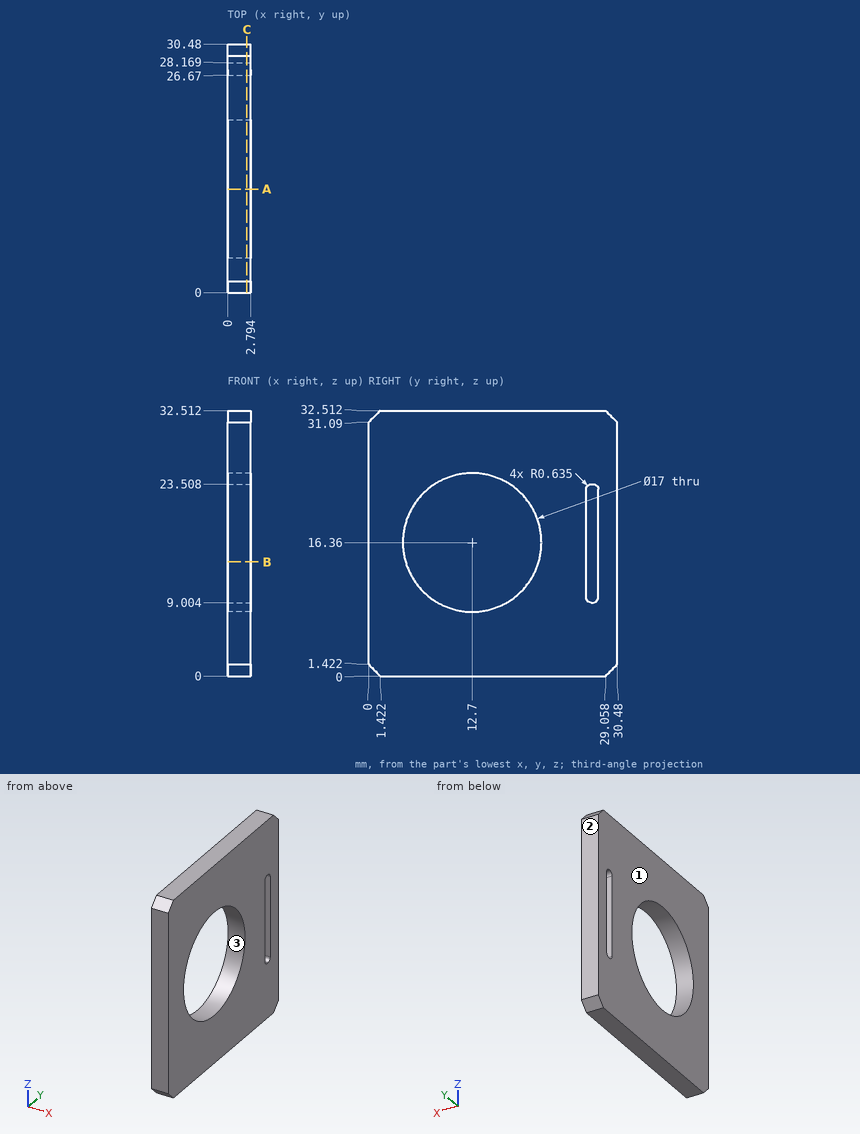
Source: three-view drawing plus pictorial views. Frame: mm from the lowest corner of the part. Round coordinates to 2 decimals unless told otherwise and drop trailing zeros. Loops run counter-clockwise (first coordinate to the right, second up) from the corner with the lowest first, then second, coordinate; pieces in that order, holes last. Notation, with made-up numbers: M 16,-35.75 L 38,-35.75 A28 cw 38,2.25 Z; hole C 14,2.5 d4. An arc over 180 degrees is marked long. Answer as CSV lines item,"result". Start each with the question number.
(1) Section B-B, the plane z = 14. Output: boundary loops of the cut face in (x, y).
(2) Draft query along Y for the marked faces 1, 2 and 3. Return one class per face: released by +Y, released by -Y, zero draft, split by the parting line, or undercut.
(3) First-contact query: pin 1 (1.5 mm diameter, centred on y = 12.5, z = 23, fed in from -X). Flat tip, straight axial feed; report the tip coordinate or a pass-through.
(4) Section A-A, the plane y = 12.7. Output: boundary loops of the cut face in (x, z).
(5) Line query: line 1 (Y direction, x = 1.95, z = 16.5); line 2 (Z direction, x = 2, y = 12.7); line 3 (Y direction, x = 0.75, z = 20). Output: solid intervals per line, ascending. Write a range as [from, to].
(6) Section C-C, the plane x = 2.35. State how many separate pieces and enclosed holes the cut face has.
Values found:
1,outline,"M 0,0 L 2.79,0 L 2.79,4.53 L 0,4.53 Z; M 0,20.87 L 2.79,20.87 L 2.79,26.67 L 0,26.67 Z; M 0,28.17 L 2.79,28.17 L 2.79,30.48 L 0,30.48 Z"
2,face 1,"zero draft"
2,face 2,"released by +Y"
2,face 3,"undercut"
3,pin 1,"passes through"
4,outline,"M 0,0 L 2.79,0 L 2.79,7.86 L 0,7.86 Z; M 0,24.86 L 2.79,24.86 L 2.79,32.51 L 0,32.51 Z"
5,line 1,"y = [0, 4.2], [21.2, 26.67], [28.17, 30.48]"
5,line 2,"z = [0, 7.86], [24.86, 32.51]"
5,line 3,"y = [0, 5.02], [20.38, 26.67], [28.17, 30.48]"
6,separate pieces,"1"
6,enclosed holes,"2"
